The listing builds one solid part. Answer for the finished solid, in the listing's coordinates (mm). A direction names the side the tool comes from. Give positions to 0.01 mm unless a question says otherwise; leave off trailing zeros. Write each loop counter-clockwise with the first axis right and the second up, starting at its lowest first coordinate (ties: lowest second). Pieces come first, ordered by that corner, then holes. Notation, with made-up numbers: (-23, -26.5) - (12, -26.5) arc R22 ccw to (12, -5.5) - close; hole circle Ø8 at (-27.5, 85). An arc over 180 degrees is marked (long way). Answer in a Markdown table with one row per item. Add a question column.
from build123d import *

# Parameters (mm, degrees)
BOSS_EXTRU_1_DEPTH = 0.8
EMPREINTE1_DEPTH   = 0.8


# Read off the part's stored shape, not the designer's step: Empreinte1
with BuildPart() as part:
    # Esquisse1 → Boss.-Extru.1 (new body)
    with BuildSketch(Plane.XY):
        with BuildLine():
            Line((13.976920297, 8.69285333), (15.248093696, 6.198035062))
            ThreePointArc((15.248093696, 6.198035062), (15.422690555, 6.048915257), (15.651592804, 6.066930255))
            Line((15.651592804, 6.066930255), (17.741248134, 7.131662826))
            ThreePointArc((17.741248134, 7.131662826), (17.984943021, 7.144439851), (18.1575097, 6.971896548))
            ThreePointArc((18.1575097, 6.971896548), (19.45, 0), (18.1575097, -6.971896548))
            ThreePointArc((18.1575097, -6.971896548), (17.984943021, -7.144439851), (17.741248134, -7.131662826))
            Line((17.741248134, -7.131662826), (15.651592804, -6.066930255))
            ThreePointArc((15.651592804, -6.066930255), (15.422690555, -6.048915257), (15.248093696, -6.198035062))
            Line((15.248093696, -6.198035062), (13.976920297, -8.69285333))
            ThreePointArc((13.976920297, -8.69285333), (13.958905299, -8.921755578), (14.108025104, -9.096352437))
            Line((14.108025104, -9.096352437), (16.197680434, -10.161085008))
            ThreePointArc((16.197680434, -10.161085008), (16.351257526, -10.350728166), (16.313099211, -10.591755952))
            ThreePointArc((16.313099211, -10.591755952), (-19.45, 0), (16.313099211, 10.591755952))
            ThreePointArc((16.313099211, 10.591755952), (16.351257526, 10.350728166), (16.197680434, 10.161085008))
            Line((16.197680434, 10.161085008), (14.108025104, 9.096352437))
            ThreePointArc((14.108025104, 9.096352437), (13.958905299, 8.921755578), (13.976920297, 8.69285333))
        make_face()
    extrude(amount=BOSS_EXTRU_1_DEPTH)

    # Empreinte1 outline → Empreinte1 (cut)
    with BuildSketch(Plane.XY):
        with BuildLine():
            ThreePointArc((9.2092, 1.678974794), (8.977813151, 2.650885141), (8.644162553, 3.5926))
            Line((8.644162553, 3.5926), (2.470606857, 7.337))
            ThreePointArc((2.470606857, 7.337), (0, 7.7418), (-2.470606857, 7.337))
            Line((-2.470606857, 7.337), (-8.644162553, 3.5926))
            ThreePointArc((-8.644162553, 3.5926), (-8.977813151, 2.650885141), (-9.2092, 1.678974794))
            Line((-9.2092, 1.678974794), (-9.2092, -1.678974794))
            ThreePointArc((-9.2092, -1.678974794), (-8.977813151, -2.650885141), (-8.644162553, -3.5926))
            Line((-8.644162553, -3.5926), (-3.388297568, -6.7804))
            Line((-3.388297568, -6.7804), (3.388297568, -6.7804))
            Line((3.388297568, -6.7804), (8.644162553, -3.5926))
            ThreePointArc((8.644162553, -3.5926), (8.977813151, -2.650885141), (9.2092, -1.678974794))
            Line((9.2092, -1.678974794), (9.2092, 1.678974794))
        make_face()
    extrude(amount=EMPREINTE1_DEPTH, mode=Mode.SUBTRACT)


solid = part.part
1. Section B-B (y = 0) is taken. Give the vertices of the cut face in (x, z), and give its area (3 significant figures).
2. The mould has two halves that part along Y. Classify faces 4 (the face through (19.45, 0.1, 0.39)), 5 (the face through (0, -8, 0)), 6 (the face through (14.604, 7.463, 0.394)), 7 (the face through (-5.5, 5.5, 0.4)): +Y half, -Y half, draft (parallel to the pull), parting line (faces both ways), or undercut.
3. Section D-D (y = -17) is taken. Give the vertices of the cut face in (x, z).
4. Straight lines are drawn through the part: L1, parallel to X at y = 0, z = 0.15; L2, parallel to Y at x = 15, z = 0.15; L3, parallel to Y at x = -1.5, z = 0.35. For each, find the intervals that lie inside material, in ascending order. Write a range as [from, to].
5. Section A-A (x = 0) is taken. Give the vertices of the cut face in (y, z), and give its area (3 significant figures).
6. A tool of negligible diameter and unlimited length cuts with its end or side. For faces 1 (the face through (15.1, -9.6, 0.4)), 2 (the face through (0, -8, 0.8)), 3 (the face through (-6.053, -5.164, 0.394)), from which of +Z, -Z, +X, -X, +Y, -Y can it reach the whole face along a straight path? Write none if from no direction.
7. Section C-C (z = 0.4) is taken. Give the vertices of the cut face in (x, y).
Geometry check:
| question | item | result |
|---|---|---|
| 1 | outline | (-19.45, 0) - (-9.21, 0) - (-9.21, 0.8) - (-19.45, 0.8) - close; (9.21, 0) - (19.45, 0) - (19.45, 0.8) - (9.21, 0.8) - close |
| 1 | area | 16.4 mm² |
| 2 | face 4 | parting line |
| 2 | face 5 | draft |
| 2 | face 6 | undercut |
| 2 | face 7 | undercut |
| 3 | outline | (-9.45, 0) - (9.45, 0) - (9.45, 0.8) - (-9.45, 0.8) - close |
| 4 | L1 | [-19.45, -9.21], [9.21, 19.45] |
| 4 | L2 | [-12.38, -9.55], [-6.68, 6.68], [9.55, 12.38] |
| 4 | L3 | [-19.39, -6.78], [7.6, 19.39] |
| 5 | outline | (-19.45, 0) - (-6.78, 0) - (-6.78, 0.8) - (-19.45, 0.8) - close; (7.74, 0) - (19.45, 0) - (19.45, 0.8) - (7.74, 0.8) - close |
| 5 | area | 19.5 mm² |
| 6 | face 1 | +Z, -Z, +X |
| 6 | face 2 | +Z, +X, -X, +Y, -Y |
| 6 | face 3 | +Z, -Z |
| 7 | outline | (13.98, -8.69) - (15.25, -6.2) arc R0.3 cw to (15.65, -6.07) - (17.74, -7.13) arc R0.3 ccw to (18.16, -6.97) arc R19.45 ccw to (18.16, 6.97) arc R0.3 ccw to (17.74, 7.13) - (15.65, 6.07) arc R0.3 cw to (15.25, 6.2) - (13.98, 8.69) arc R0.3 cw to (14.11, 9.1) - (16.2, 10.16) arc R0.3 ccw to (16.31, 10.59) arc R19.45 ccw (long way) to (16.31, -10.59) arc R0.3 ccw to (16.2, -10.16) - (14.11, -9.1) arc R0.3 cw to start; hole (-9.21, -1.68) arc R9.36 ccw to (-8.64, -3.59) - (-3.39, -6.78) - (3.39, -6.78) - (8.64, -3.59) arc R9.36 ccw to (9.21, -1.68) - (9.21, 1.68) arc R9.36 ccw to (8.64, 3.59) - (2.47, 7.34) arc R7.74 ccw to (-2.47, 7.34) - (-8.64, 3.59) arc R9.36 ccw to (-9.21, 1.68) - close |
